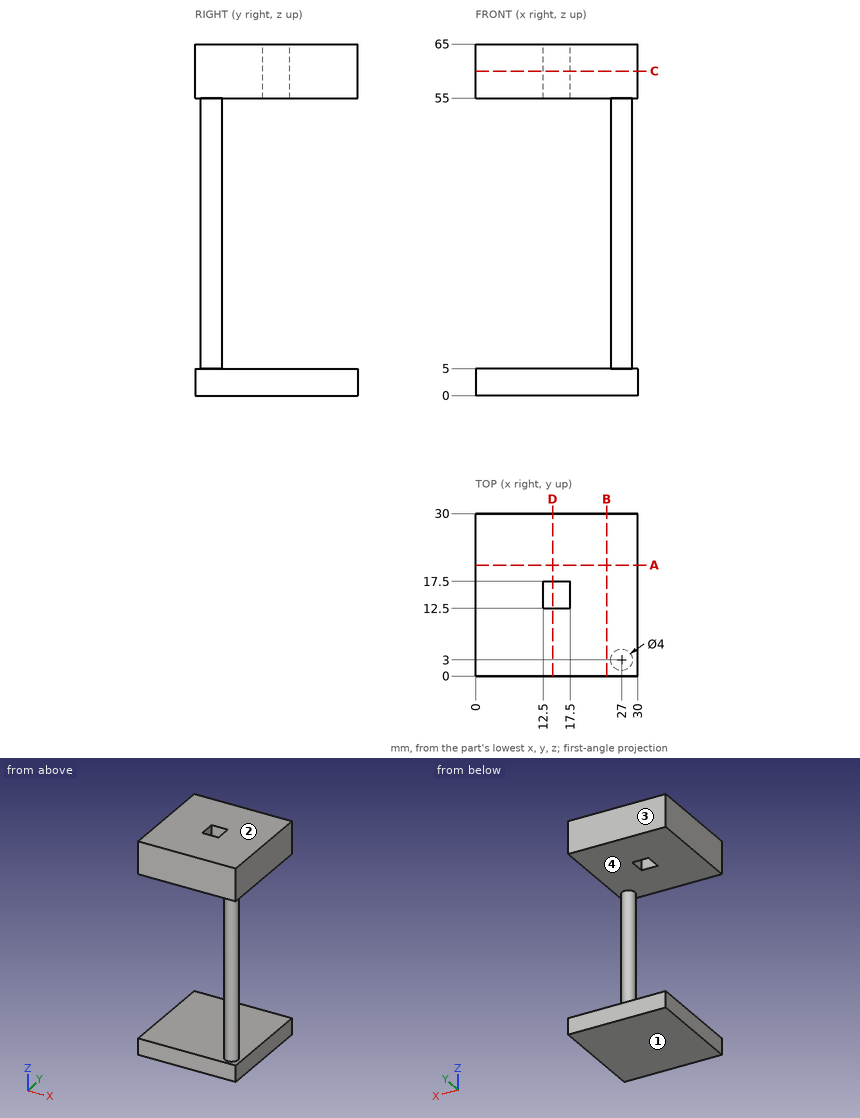
Input: dimensioned drawing with shaded views. Units: mm. Origin: part minimum x, y, z. Give positions to 0.01 mm unless a question says otherwise; leave off trailing zeros. Order: outer loops, then holes, each group sorted by start corner. A loop starts at its lowest first (then second) coordinate and runs counter-clockwise, first axis right, second up. Notation, with made-up numbers: (30.5, 10.25) -> (77.5, 10.25) arc R16 ccw to (77.5, 36.25) -> close; hole circle Ø2 at (-14.5, 23.5). An arc over 180 degrees is marked (long way). Use a Markdown table: item, result.
1) Section query C-C, the plane z = 60. Return the cut outline in (x, y).
Answer list:
| item | result |
|---|---|
| outline | (0, 0) -> (30, 0) -> (30, 30) -> (0, 30) -> close; hole (12.5, 12.5) -> (17.5, 12.5) -> (17.5, 17.5) -> (12.5, 17.5) -> close |
2) Ray query, line 1 along Z through (x, y) = (10.25, 9.5); line 2 along X through (y, z) = (4, 29). Return the intervals inside material, ascending. Write a range as [from, to].
Answer list:
| item | result |
|---|---|
| line 1 | [0, 5], [55, 65] |
| line 2 | [25.27, 28.73] |
3) Section query D-D, the plane x = 14.25. Return the cut outline in (y, z).
Answer list:
| item | result |
|---|---|
| outline | (0, 0) -> (30, 0) -> (30, 5) -> (0, 5) -> close; (0, 55) -> (12.5, 55) -> (12.5, 65) -> (0, 65) -> close; (17.5, 55) -> (30, 55) -> (30, 65) -> (17.5, 65) -> close |
4) Mould query, pull axis Z, two halves, no side actions, for the marked faces 1, 2, 3 and 4. Classes: +Z half, -Z half, draft (parallel to the pull), parting line (faces both ways), or undercut.
Answer list:
| item | result |
|---|---|
| face 1 | -Z half |
| face 2 | +Z half |
| face 3 | draft |
| face 4 | undercut |
5) Section query A-A, the plane y = 20.5. Return the cut outline in (x, z).
Answer list:
| item | result |
|---|---|
| outline | (0, 0) -> (30, 0) -> (30, 5) -> (0, 5) -> close; (0, 55) -> (30, 55) -> (30, 65) -> (0, 65) -> close |
6) Contact query for flat-ended pins moving along their axis: P1, Ø12, axis at x = 17, z = 51.5, coming from the -Y side; P2, Ø5, axis at y = 5.5, z = 41, coming from the -X side. Output: stop coordinate, or through.
Answer list:
| item | result |
|---|---|
| P1 | y = 0 |
| P2 | x = 25 |
